```python
from build123d import *

# Parameters (mm, degrees)
SKETCH1_RX          = 38.1
SKETCH1_RY          = 21.209
BOSS_EXTRUDE1_DEPTH = 6.35
CUT_EXTRUDE6_DEPTH  = 45.065339906
CUT_EXTRUDE8_DEPTH  = 3.81
BOSS_EXTRUDE2_DEPTH = 11.938
CUT_EXTRUDE11_DEPTH = 45.310625914
CUT_EXTRUDE10_DEPTH = 6.35
CUT_EXTRUDE14_START = -6.35
SKETCH16_W          = 7.366
SKETCH16_H          = 5.8166
CUT_EXTRUDE14_DEPTH = 6.35


with BuildPart() as part:
    # Sketch1 → Boss-Extrude1 (new body)
    with BuildSketch(Plane(origin=(0, 0, 0), x_dir=(1, 0, 0), z_dir=(0, 1, 0))):
        with Locations(Location((0, 0), (0, 0, 90))):
            Ellipse(SKETCH1_RX, SKETCH1_RY)
    extrude(amount=BOSS_EXTRUDE1_DEPTH)

    # Sketch7 → Cut-Extrude6 (cut, through all)
    with BuildSketch(Plane(origin=(0, 6.35, 0), x_dir=(1, 0, 0), z_dir=(0, 1, 0))):
        with BuildLine():
            Line((-11.723715863, 31.75), (11.723715863, 31.75))
            add(Edge.make_bspline(
                [(11.723715863, 31.75), (0, 45.72), (-11.723715863, 31.75)],
                knots=[5.697499764, 5.697499764, 5.697499764, 6.868870851, 6.868870851, 6.868870851], degree=2, weights=[1, 0.833333333, 1]))
        make_face()
    extrude(amount=-CUT_EXTRUDE6_DEPTH, mode=Mode.SUBTRACT)

    # Sketch8 → Cut-Extrude8 (cut)
    with BuildSketch(Plane.XZ):
        Polygon((5.969, -31.75), (5.969, -24.1554), (25.250257638, -24.1554), (25.250257638, -46.762779547), (-25.868253854, -46.762779547), (-25.868253854, -24.1554), (-5.969, -24.1554), (-5.969, -31.75), align=None)
    extrude(amount=-CUT_EXTRUDE8_DEPTH, mode=Mode.SUBTRACT)

    # Sketch9 → Boss-Extrude2 (add)
    with BuildSketch(Plane(origin=(5.969, 0, 0), x_dir=(0, 0, -1), z_dir=(1, 0, 0))):
        Polygon((24.1554, 3.81), (24.1554, -2.032), (24.257, -2.032), (27.305, -4.064), (31.75, -4.064), (31.75, 3.81), align=None)
    extrude(amount=-BOSS_EXTRUDE2_DEPTH)

    # Sketch10 → Cut-Revolve1 (revolve, cut)
    with BuildSketch(Plane(origin=(5.969, 0, 0), x_dir=(0, 0, -1), z_dir=(1, 0, 0))):
        with BuildLine():
            Line((28.0162, -0.635), (28.0162, 0.635))
            ThreePointArc((28.0162, 0.635), (28.6512, 0), (28.0162, -0.635))
        make_face()
    cut_revolve1 = revolve(axis=Axis((5.969, -0.635, -28.0162), (0, 1, 0)), mode=Mode.SUBTRACT)

    # Sketch14 → Cut-Revolve2 (revolve, cut)
    with BuildSketch(Plane(origin=(0, 0, 0), x_dir=(-1, 0, 0), z_dir=(0, -1, 0))):
        Polygon((-5.969, 25.6667), (-4.064, 25.9842), (-4.064, 28.0162), (-5.969, 28.0162), align=None)
    cut_revolve2 = revolve(axis=Axis((-0.604514271, 0, -28.0162), (1, 0, 0)), mode=Mode.SUBTRACT)

    # Sketch13 → Cut-Extrude11 (cut, through all)
    with BuildSketch(Plane.XZ.offset(-3.81)):
        with BuildLine():
            Line((16.401620572, -24.1554), (5.969, -24.1554))
            Line((5.969, -24.1554), (5.969, -31.75))
            Line((5.969, -31.75), (11.723715863, -31.75))
            add(Edge.make_bspline(
                [(11.723715863, -31.75), (14.380408678, -28.584280269), (16.401620572, -24.1554)],
                knots=[0.585685543, 0.585685543, 0.585685543, 0.884081597, 0.884081597, 0.884081597], degree=2, weights=[1, 0.988890605, 1]))
        make_face()
        with BuildLine():
            Line((-11.723715863, -31.75), (-5.969, -31.75))
            Line((-5.969, -31.75), (-5.969, -24.1554))
            Line((-5.969, -24.1554), (-16.401620572, -24.1554))
            add(Edge.make_bspline(
                [(-16.401620572, -24.1554), (-14.380408678, -28.584280269), (-11.723715863, -31.75)],
                knots=[5.39910371, 5.39910371, 5.39910371, 5.697499764, 5.697499764, 5.697499764], degree=2, weights=[1, 0.988890605, 1]))
        make_face()
    extrude(amount=-CUT_EXTRUDE11_DEPTH, mode=Mode.SUBTRACT)

    # Sketch12 → Cut-Extrude10 (cut)
    with BuildSketch(Plane(origin=(0, 6.35, -25.4), x_dir=(-1, 0, 0), z_dir=(0, -1, 0))):
        Polygon((-5.969, 0.2667), (-4.445, 0.7747), (-4.445, 4.4577), (-5.969, 4.9657), align=None)
    cut_extrude10 = extrude(amount=CUT_EXTRUDE10_DEPTH, mode=Mode.SUBTRACT)

    # Mirror1: Cut-Revolve1, Cut-Revolve2, Cut-Extrude10 across plane
    add(cut_revolve1.mirror(Plane(origin=(0, 0, 0), x_dir=(0, 0, 1), z_dir=(1, 0, 0))), mode=Mode.SUBTRACT)
    add(cut_revolve2.mirror(Plane(origin=(0, 0, 0), x_dir=(0, 0, 1), z_dir=(1, 0, 0))), mode=Mode.SUBTRACT)
    add(cut_extrude10.mirror(Plane(origin=(0, 0, 0), x_dir=(0, 0, 1), z_dir=(1, 0, 0))), mode=Mode.SUBTRACT)

    # Sketch16 → Cut-Extrude14 (cut)
    with BuildSketch(Plane(origin=(0, 6.35, 0), x_dir=(1, 0, 0), z_dir=(0, 1, 0)).offset(CUT_EXTRUDE14_START)):
        with Locations((0, 27.8257)):
            Rectangle(SKETCH16_W, SKETCH16_H)
    extrude(amount=CUT_EXTRUDE14_DEPTH, mode=Mode.SUBTRACT)


solid = part.part
```
Input: part model. Units: mm. Frame: model coordinates. A direction names the side the tool comes from. Coordinates: 2 decimals unless noted, no trailing zeros. One line per item, written item: value.
(1) Line query: line 1 along X through (y, z) = (5, -27) (3 decimals); line 2 along Y through (x, z) = (-16.5, -19.5); line 3 along Z through (x, y) = (5, 1). Output: solid intervals per line, ascending. Write a range as from..to.
Filled in:
line 1: -4.445..-3.683, 3.683..4.445
line 2: 0..6.35
line 3: -31.75..-30.04, -25.99..37.03
(2) Reachability of faces 1 (the flat face through (-5.218, 3.219, -25.917)), 2 (the flat face through (-4.064, 0, -28)), 3 (the flat face through (5.218, 3.219, -25.917)), 4 (the flat face through (3.683, 3, -28)) from +Z, -Z, +X, -X, +Y, -Y: full face, straight path, thin tool, end or side. Return the list, or none.
Filled in:
face 1: -X, +Y
face 2: -X
face 3: +X, +Y
face 4: +Y
(3) Pin query (flat end, axial travel): pin 1 (1.2 mm diameter, centred on y = 0.5, z = -28.5, fed in from -X); pin 2 (3 mm diameter, centred on x = 9, y = 2.5, fed in from -Z); pin 3 (4.5 mm diameter, centred on y = -1, z = -27.5, fed in from +X). Return the tip coordinate at first contact, or that it passes through.
Filled in:
pin 1: x = -4.06
pin 2: z = -24.16
pin 3: x = 5.97
(4) Pull-direction query (Z, two-part tool) for faces 5 (the flat face through (0.084, -3.034, -25.76)), 6 (the flat face through (-5.2, 3.22, -30.11)), 7 (the flat face through (-11, 3, -24.155)), 8 (the flat face through (4.445, 4, -28)); classes: +Z half, -Z half, draft (parallel to the pull), parting line (faces both ways), or undercut.
Filled in:
face 5: +Z half
face 6: undercut
face 7: -Z half
face 8: undercut
